Can you work these out from the model? Positions are in its coordinate system, mm. A direction names the side the tool comes from. Give positions to 0.01 mm unless a question says otherwise; leave off trailing zeros. Loops run counter-clockwise (first coordinate to the right, second up) from the corner with the lowest first, then second, coordinate; pieces in that order, holes last. Notation, with made-up numbers: (76, 3.25) - (88, 3.25) arc R19 ccw to (88, 19.25) - close; hole circle Ø7 at (12, 56). An arc over 180 degrees is marked (long way). Write item = value, one per line.
from build123d import *

# Parameters (mm, degrees)
SKETCH2_W            = 150
SKETCH2_H            = 40
BOSS_EXTRUDE1_DEPTH  = 10
FILLET2_R            = 20
SKETCH10_W           = 50
SKETCH10_H           = 10
BOSS_EXTRUDE4_DEPTH  = 55
SKETCH12_R           = 15
CUT_EXTRUDE2_DEPTH   = 10
FILLET3_R            = 25
FILLET3_OF_MIRROR1_R = 25
FILLET4_R            = 20
CUT_EXTRUDE4_DEPTH   = 10


with BuildPart() as part:
    # Sketch2 → Boss-Extrude1 (new body)
    with BuildSketch(Plane(origin=(0, 0, 0), x_dir=(1, 0, 0), z_dir=(0, 1, 0))):
        Rectangle(SKETCH2_W, SKETCH2_H)
    boss_extrude1 = extrude(amount=BOSS_EXTRUDE1_DEPTH)

    # Fillet2
    fillet2_edges = [part.edges().sort_by_distance(p)[0] for p in [
        (-75, 5, 20),
        (-75, 5, -20),
    ]]
    fillet(fillet2_edges, radius=FILLET2_R - 0.0001)  # a hair under: the kernel refuses the full size

    # Sketch10 → Boss-Extrude4 (add)
    with BuildSketch(Plane(origin=(0, 10, 0), x_dir=(1, 0, 0), z_dir=(0, 1, 0))):
        with Locations((50, -15)):
            Rectangle(SKETCH10_W, SKETCH10_H)
    boss_extrude4 = extrude(amount=BOSS_EXTRUDE4_DEPTH)

    # Sketch12 → Cut-Extrude2 (cut)
    with BuildSketch(Plane.XY.offset(20)):
        with Locations((50, 40)):
            Circle(SKETCH12_R)
    cut_extrude2 = extrude(amount=-CUT_EXTRUDE2_DEPTH, mode=Mode.SUBTRACT)

    # Fillet3
    fillet3_edges = [part.edges().sort_by_distance(p)[0] for p in [
        (75, 65, 15),
        (25, 65, 15),
    ]]
    fillet(fillet3_edges, radius=FILLET3_R - 0.0001)  # a hair under: the kernel refuses the full size

    # Mirror1: Boss-Extrude1, Boss-Extrude4 across plane
    add(boss_extrude1.mirror(Plane.XY))
    add(boss_extrude4.mirror(Plane.XY))

    # Fillet3 of Mirror1
    fillet3_of_mirror1_edges = [part.edges().sort_by_distance(p)[0] for p in [
        (75, 65, -15),
        (25, 65, -15),
    ]]
    fillet(fillet3_of_mirror1_edges, radius=FILLET3_OF_MIRROR1_R - 0.0001)  # a hair under: the kernel refuses the full size

    # Mirror2: Cut-Extrude2 across plane
    add(cut_extrude2.mirror(Plane.XY), mode=Mode.SUBTRACT)

    # Fillet4
    fillet4_edges = [part.edges().sort_by_distance(p)[0] for p in [
        (-75, 5, -20),
        (-75, 5, 20),
    ]]
    fillet(fillet4_edges, radius=FILLET4_R - 0.0001)  # a hair under: the kernel refuses the full size

    # Sketch9 → Cut-Extrude4 (cut)
    with BuildSketch(Plane(origin=(0, 10, 0), x_dir=(1, 0, 0), z_dir=(0, 1, 0))):
        with BuildLine():
            Line((-55, 10), (-15, 10))
            ThreePointArc((-15, 10), (-5, 0), (-15, -10))
            Line((-15, -10), (-55, -10))
            ThreePointArc((-55, -10), (-65, 0), (-55, 10))
        make_face()
    extrude(amount=-CUT_EXTRUDE4_DEPTH, mode=Mode.SUBTRACT)


solid = part.part
Q1. I need wall thicknesses on L1, parallel to Y at x = 50, z = 16; L2, parallel to Z at x = 37.5, y = 13; L3, parallel to X at y = 16.5, z = 18. Which ranges of each line are inside material? Lowest first, please.
Output:
L1 = 0 to 25, 55 to 65
L2 = -20 to -10, 10 to 20
L3 = 25 to 75
Q2. Which directions (+Z, -Z, +X, -X, +Y, -Y) give clear straight access to the entire face, cutting with the end or side of a thin tool? Please do faces 5 (the flat face through (44, 25, -10)), 6 (the flat face through (25, 25, 15)), 7 (the flat face through (-35, 5, 10)).
Output:
face_5 = +X, -X, +Y
face_6 = +Z, -Z, -X, +Y
face_7 = +Y, -Y
Q3. We'd pull the mould along Y, two halves only. Please class faces 1 (the cylindrical face through (38.944, 50.138, -15.07)), 2 (the flat face through (16, 0, 0)), 3 (the cylindrical face through (38.944, 50.138, 15.07)), 4 (the flat face through (-1, 10, 0)): released by +Y, released by -Y, zero draft, split by the parting line, or undercut.
Output:
face_1 = undercut
face_2 = released by -Y
face_3 = undercut
face_4 = released by +Y
Q4. For pin 1 (10 mm diameter, centred on x = -36.5, z = -15, fed in from +Y); pin 2 (8 mm diameter, centred on y = 32.5, z = 16.5, fed in from -X); pin 3 (5 mm diameter, centred on y = 53.5, z = -13, fed in from +X), each with a flat end and sliding along its axis, tell me the tip position at first contact or that it passes through.
Output:
pin_1 = 10
pin_2 = 25
pin_3 = 72.45
Q5. Imagine slicing it at A-A, the plane y = 18.5. Write out the boundary of the cut face in (x, z).
Output:
outline = (25, -20) - (75, -20) - (75, -10) - (25, -10) - close; (25, 10) - (75, 10) - (75, 20) - (25, 20) - close
Q6. Imagine slicing it at D-D, the plane y = 28.5. Write out the boundary of the cut face in (x, z), then the cut area to 3 significant figures.
Output:
outline = (25, -20) - (40.37, -20) - (40.37, -10) - (25, -10) - close; (25, 10) - (40.37, 10) - (40.37, 20) - (25, 20) - close; (59.63, -20) - (75, -20) - (75, -10) - (59.63, -10) - close; (59.63, 10) - (75, 10) - (75, 20) - (59.63, 20) - close
area = 615 mm2
Q7. Imagine slicing it at B-B, the plane x = -20. Write out the boundary of the cut face in (y, z), then the cut area to 3 significant figures.
Output:
outline = (0, -20) - (10, -20) - (10, -10) - (0, -10) - close; (0, 10) - (10, 10) - (10, 20) - (0, 20) - close
area = 200 mm2
